Geometry: see drawing. Coordinates: mm, zero at the bounding-box minimum. A direction names the side the tool comes from. Give positions to 0.01 mm unless a question says otherwise; leave off trailing zeros. Order: outer loops, then holes, each group sorted by start corner. A loop starts at its lowest first (then second) coordinate and runs counter-clockwise, first axis right, second up. Notation, with made-up numbers: (34.5, 67) - (81.5, 67) arc R17 cw to (81.5, 87) - close; hole circle Ø1 at (45.25, 18.25). An arc over 180 degrees is marked (long way). Put each result on its own line as item: value. Start each with the question number.
1. Ray query, line 1 along Z through (x, y) = (5, 14.5); line 2 along X through (y, z) = (18.75, 7.5); line 3 along Y through (x, z) = (10, 2). Return the intervals inside material, ascending. Write a range as from..to.
2. Section D-D on x = 11. Count the separate pieces of the cut face and the enclosed holes in it, plus the area to 3 significant figures.
3. Section B-B on z = 7.5. Return the cut outline in (x, y), plus the area to 3 significant figures.
4. Mould query, pull axis Z, two halves, no side actions, for the marked faces 3, 4, 5 and 6. Classes: pulls with the +Z half, pulls with the -Z half, needs draft (parallel to the pull), parting line crosses it, or undercut.
5. Section A-A on y = 13.75. Return the cut outline in (x, z), plus the area to 3 significant figures.
6. Section C-C on y = 4.75. Return the cut outline in (x, z), plus the area to 3 significant figures.
7. First-contact query: P1, Ø2, axis at x = 13, z = 6.5, coming from the +Y side; P2, Ø2.5, axis at x = 7.5, z = 7, coming from the -Y side. Flat tips, straight axial feed; report the tip coordinate or a pass-through.
8. Set-up query: the marked faces 1 and 2. Return all of +Z, -Z, +X, -X, +Y, -Y with unobstructed straight access to the full face (end or side cutting, diameter ignored); none if empty.
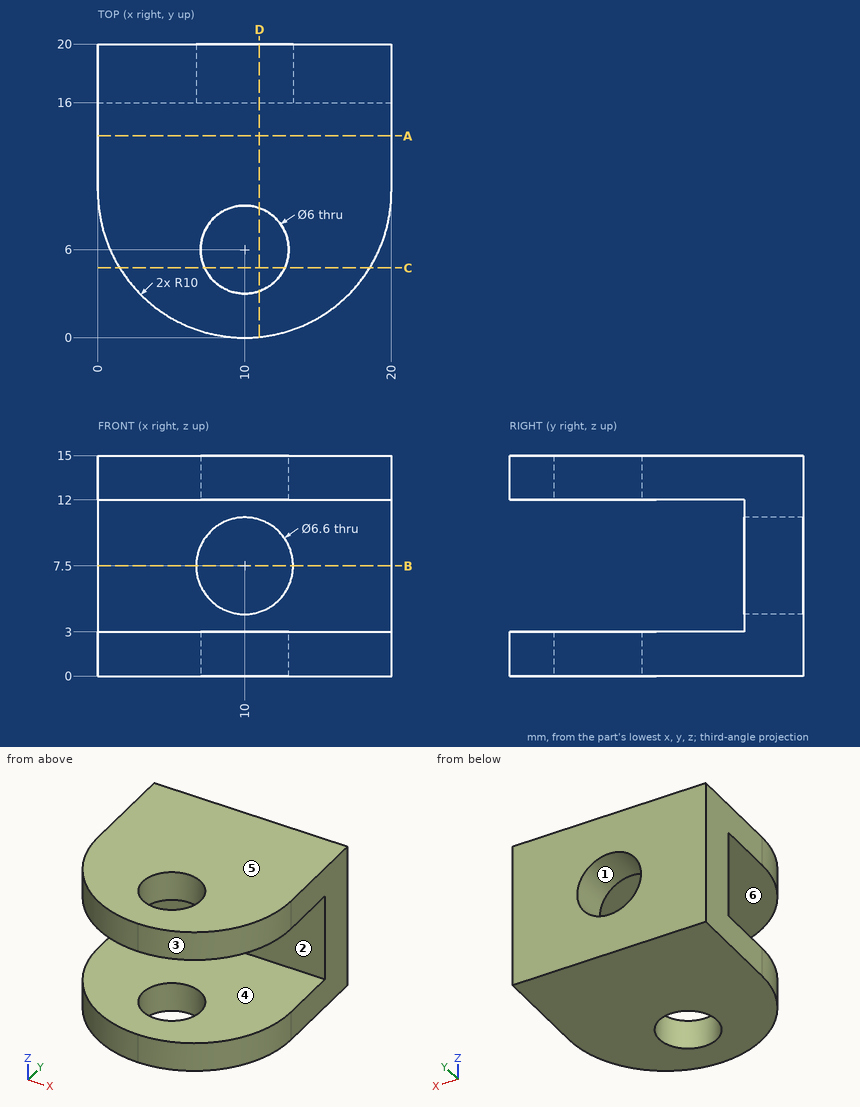
Resolved:
1. line 1: 0..3, 12..15
1. line 2: 0..6.7, 13.3..20
1. line 3: 0..3, 9..20
2. separate pieces: 4
2. enclosed holes: 0
2. area: 96.6 mm^2
3. outline: (0, 16) - (6.7, 16) - (6.7, 20) - (0, 20) - close; (13.3, 16) - (20, 16) - (20, 20) - (13.3, 20) - close
3. area: 53.6 mm^2
4. face 3: needs draft
4. face 4: undercut
4. face 5: pulls with the +Z half
4. face 6: undercut
5. outline: (0, 0) - (20, 0) - (20, 3) - (0, 3) - close; (0, 12) - (20, 12) - (20, 15) - (0, 15) - close
5. area: 120 mm^2
6. outline: (1.49, 0) - (7.27, 0) - (7.27, 3) - (1.49, 3) - close; (1.49, 12) - (7.27, 12) - (7.27, 15) - (1.49, 15) - close; (12.73, 0) - (18.51, 0) - (18.51, 3) - (12.73, 3) - close; (12.73, 12) - (18.51, 12) - (18.51, 15) - (12.73, 15) - close
6. area: 69.4 mm^2
7. P1: y = 20
7. P2: y = 16
8. face 1: +Y, -Y
8. face 2: +X, -X, -Y
